```python
from build123d import *

# Parameters (mm, degrees)
SKETCH2_W           = 5.3
SKETCH2_H           = 25
SKETCH2_R           = 1.5
BOSS_EXTRUDE1_DEPTH = 3
SKETCH3_W           = 50
SKETCH3_H           = 45
BOSS_EXTRUDE2_DEPTH = 3
SKETCH7_W           = 38.35
SKETCH7_H           = 3
BOSS_EXTRUDE3_DEPTH = 45
CUT_EXTRUDE1_DEPTH  = 5
SKETCH8_3_R         = 1.5
CUT_EXTRUDE2_DEPTH  = 5
SKETCH11_R          = 1.5
CUT_EXTRUDE4_DEPTH  = 5
SKETCH12_W          = 18.7
SKETCH12_H          = 45
BOSS_EXTRUDE4_DEPTH = 3


with BuildPart() as part:
    # Sketch2 → Boss-Extrude1 (new body)
    # profile 1 of 3: a face of its own
    with BuildSketch(Plane.XY):
        with Locations((10.025, 0)):
            Rectangle(SKETCH2_W, SKETCH2_H)
    # profile 2 of 3: a face of its own
    with BuildSketch(Plane.XY):
        Polygon((7.375, 12.5), (12.675, 12.5), (12.675, 22.5), (-12.675, 22.5), (-12.675, 12.5), align=None)
        with Locations((-1.505, 17.58)):
            Circle(SKETCH2_R, mode=Mode.SUBTRACT)
    # profile 3 of 3: a face of its own
    with BuildSketch(Plane.XY):
        Polygon((-12.675, -22.5), (12.675, -22.5), (12.675, -12.5), (7.375, -12.5), (-12.675, -12.5), align=None)
        with Locations((-10.375, -17.5)):
            Circle(SKETCH2_R, mode=Mode.SUBTRACT)
        with Locations((7.375, -17.5)):
            Circle(SKETCH2_R, mode=Mode.SUBTRACT)
    extrude(amount=-BOSS_EXTRUDE1_DEPTH)

    # Sketch3 → Boss-Extrude2 (add)
    with BuildSketch(Plane(origin=(12.675, 0, 0), x_dir=(0, 0, -1), z_dir=(1, 0, 0))):
        with Locations((25, 0)):
            Rectangle(SKETCH3_W, SKETCH3_H)
    extrude(amount=BOSS_EXTRUDE2_DEPTH)

    # Sketch7 → Boss-Extrude3 (add)
    with BuildSketch(Plane(origin=(0, 22.5, 0), x_dir=(1, 0, 0), z_dir=(0, 1, 0))):
        with Locations((-3.5, 23.2)):
            Rectangle(SKETCH7_W, SKETCH7_H)
    extrude(amount=-BOSS_EXTRUDE3_DEPTH)

    # Sketch8 → Cut-Extrude1 (cut)
    with BuildSketch(Plane.XY.offset(-21.7)):
        Polygon((-12.675, 12.572802409), (-12.675, 22.5), (-22.675, 22.5), (-22.675, -22.5), (-12.675, -22.5), (-12.675, -12.5), (7.375, -12.5), (7.375, 12.572802409), align=None)
    extrude(amount=-CUT_EXTRUDE1_DEPTH, mode=Mode.SUBTRACT)

    # Sketch8<3> → Cut-Extrude2 (cut)
    with BuildSketch(Plane.XY.offset(-21.7)):
        with Locations((-1.505, 17.58)):
            Circle(SKETCH8_3_R)
        with Locations((-10.375, -17.5)):
            Circle(SKETCH8_3_R)
        with Locations((7.375, -17.5)):
            Circle(SKETCH8_3_R)
    extrude(amount=-CUT_EXTRUDE2_DEPTH, mode=Mode.SUBTRACT)

    # Sketch11 → Cut-Extrude4 (cut)
    with BuildSketch(Plane(origin=(15.675, 0, 0), x_dir=(0, 0, -1), z_dir=(1, 0, 0))):
        with Locations((33, 14.5)):
            Circle(SKETCH11_R)
        with Locations((45, 14.5)):
            Circle(SKETCH11_R)
        with Locations((33, -12.5)):
            Circle(SKETCH11_R)
        with Locations((45, -12.5)):
            Circle(SKETCH11_R)
    extrude(amount=-CUT_EXTRUDE4_DEPTH, mode=Mode.SUBTRACT)

    # Sketch12 → Boss-Extrude4 (add)
    with BuildSketch(Plane.ZY.offset(-12.675)):
        with Locations((-12.35, 0)):
            Rectangle(SKETCH12_W, SKETCH12_H)
    extrude(amount=BOSS_EXTRUDE4_DEPTH)


solid = part.part
```
Design review of the part built by this model. Coordinates are the model's own, in mm. A direction names the side the tool comes from. Round coordinates to 2 decimals unless told otherwise and drop trailing zeros. Write each loop counter-clockwise with the first axis right and the second up, starting at its lowest first coordinate (ties: lowest second). Pieces come first, ordered by that corner, then holes. Notation, with made-up numbers: (22.5, -15) -> (58.5, -15) arc R28 cw to (58.5, 8) -> close; hole circle Ø1 at (57.25, -18). An arc over 180 degrees is marked (long way). Answer in a Markdown table with one row per item.
Q1. Take a section at C-C, the plane x = -1. State the section outline as (y, z) points.
The answers:
| item | result |
|---|---|
| outline | (-22.5, -24.7) -> (-12.5, -24.7) -> (-12.5, -21.7) -> (-22.5, -21.7) -> close; (-22.5, -3) -> (-12.5, -3) -> (-12.5, 0) -> (-22.5, 0) -> close; (12.5, -3) -> (16.17, -3) -> (16.17, 0) -> (12.5, 0) -> close; (12.57, -24.7) -> (16.17, -24.7) -> (16.17, -21.7) -> (12.57, -21.7) -> close; (18.99, -24.7) -> (22.5, -24.7) -> (22.5, -21.7) -> (18.99, -21.7) -> close; (18.99, -3) -> (22.5, -3) -> (22.5, 0) -> (18.99, 0) -> close |
Q2. Take a section at A-A, the plane y = 17.58. State the section outline as (x, z) points (3 decimals), then the cut area to 3 significant figures.
The answers:
| item | result |
|---|---|
| outline | (-12.675, -24.7) -> (-3.005, -24.7) -> (-3.005, -21.7) -> (-12.675, -21.7) -> close; (-12.675, -3) -> (-3.005, -3) -> (-3.005, 0) -> (-12.675, 0) -> close; (-0.005, -24.7) -> (12.675, -24.7) -> (12.675, -50) -> (15.675, -50) -> (15.675, 0) -> (-0.005, 0) -> (-0.005, -3) -> (9.675, -3) -> (9.675, -21.7) -> (-0.005, -21.7) -> close |
| area | 340 mm² |
Q3. To check wall thickness, follow L1, parallel to Y at x = -1.5, z = -22.5; L2, parallel to Y at x = 13.5, z = -33; L3, parallel to Z at x = 0, y = 14. State the ranges of each line that lie inside material, in increasing order. Write a range as [from, to].
The answers:
| item | result |
|---|---|
| L1 | [-22.5, -12.5], [12.57, 16.08], [19.08, 22.5] |
| L2 | [-22.5, -14], [-11, 13], [16, 22.5] |
| L3 | [-24.7, -21.7], [-3, 0] |
Q4. Clearance check with flat-ended pins moving along their axes: pin 1 Ø3.5 at (y, z) = (-12.5, -45) entering from -X (3 decimals); pin 2 Ø2.5 at (x, y) = (7.375, -17.5) entering from -Z; pin 3 Ø2.5 at (y, z) = (5.5, -1.5) entering from -X (3 decimals); pin 4 Ø9.5 at (y, z) = (2.5, -8.5) entering from -X (3 decimals). State where each tip first meets the part, or that it passes through.
The answers:
| item | result |
|---|---|
| pin 1 | x = 12.675 |
| pin 2 | through |
| pin 3 | x = 7.375 |
| pin 4 | x = 9.675 |
Q5. For faces 4 (the face through (7.375, 0, -1)), 5 (the face through (-3, 12.573, -23)), 6 (the face through (8, 0, -3)), list the 3-axis set-ups (+Z, -Z, +X, -X, +Y, -Y) from which the entire face can be reached by the end or side of a thin tool; tool diameter is ignored.
The answers:
| item | result |
|---|---|
| face 4 | +Z, -Z, -X |
| face 5 | -Z, -X |
| face 6 | -X, +Y, -Y |
Q6. Take a section at D-D, the plane z = -45. State the section outline as (x, y) points (3 decimals).
The answers:
| item | result |
|---|---|
| outline | (12.675, -22.5) -> (15.675, -22.5) -> (15.675, -14) -> (12.675, -14) -> close; (12.675, -11) -> (15.675, -11) -> (15.675, 13) -> (12.675, 13) -> close; (12.675, 16) -> (15.675, 16) -> (15.675, 22.5) -> (12.675, 22.5) -> close |
Q7. Take a section at B-B, the plane z = -24. State the section outline as (x, y) points (3 decimals).
The answers:
| item | result |
|---|---|
| outline | (-12.675, -22.5) -> (15.675, -22.5) -> (15.675, 22.5) -> (-12.675, 22.5) -> (-12.675, 12.573) -> (7.375, 12.573) -> (7.375, -12.5) -> (-12.675, -12.5) -> close; hole circle Ø3 at (-10.375, -17.5); hole circle Ø3 at (-1.505, 17.58); hole circle Ø3 at (7.375, -17.5) |
Q8. Draft analysis for pull direction X (two halves, no side actions). For faces 1 (the face through (-1.83, 16.116, -23.179)), 2 (the face through (-3, -12.5, -23)), 3 (the face through (-12.675, 18, -1)), state which applies: +X half, -X half, draft (parallel to the pull), parting line (faces both ways), or undercut.
The answers:
| item | result |
|---|---|
| face 1 | undercut |
| face 2 | draft |
| face 3 | -X half |
